Autodesk Inventor part; units mm, degrees
ref_plane "YZ Plane" through (0, 0, 0) normal (1, 0, 0) x (0, 1, 0)
ref_plane "XZ Plane" through (0, 0, 0) normal (0, 1, 0) x (-1, 0, 0)
ref_plane "XY Plane" through (0, 0, 0) normal (0, 0, 1) x (1, 0, 0)
sketch "Sketch3" plane through (0, 0, 0) normal (0, 0, 1) x (1, 0, 0)
  line L0 (0, 25.4) -> (0, -25.4)
  line L1 (0, 25.4) -> (19.05, 25.4)
  line L2 (19.05, 25.4) -> (19.05, 22.225)
  line L3 (19.05, 22.225) -> (3.048, 22.225)
  line L4 (3.048, 22.225) -> (3.048, -22.225)
  line L5 (3.048, -22.225) -> (19.05, -22.225)
  line L6 (19.05, -22.225) -> (19.05, -25.4)
  line L7 (19.05, -25.4) -> (0, -25.4)
  line L8 (0, 0) -> (3.048, 0) construction
  dimension "d7" = 50.8
  dimension "d10" = 19.05
  dimension "d19" = 3.175
  dimension "d20" = 16.002
extrude "Extrusion3" add sketch "Sketch3" along normal mid plane 209.296
fillet "Fillet1" radius 3.175 4 edges at (19.05, 22.225, 0) (19.05, -22.225, 0) (3.048, -22.225, 0) (3.048, 22.225, 0)
sketch "Sketch4" plane through (0, -25.4, 104.648) normal (-1, 0, 0) x (0, 0, 1)
  line L0 (0, 50.8) -> (-209.296, 50.8)
  line L1 (-209.296, 50.8) -> (-193.294, 50.8)
  line L2 (-193.294, 50.8) -> (-193.294, 47.625)
  line L3 (-193.294, 47.625) -> (-209.296, 47.625)
  line L4 (-209.296, 47.625) -> (-209.296, 50.8)
  line L5 (0, 44.45) -> (-209.296, 44.45)
  line L6 (-209.296, 6.35) -> (0, 6.35)
  line L7 (-209.296, 0) -> (0, 0)
  line L8 (-209.296, 0) -> (0, 0)
  line L9 (-209.296, 0) -> (-193.294, 0)
  line L10 (-193.294, 0) -> (-193.294, 3.175)
  line L11 (-193.294, 3.175) -> (-209.296, 3.175)
  line L12 (-209.296, 3.175) -> (-209.296, 0)
  line L13 (0, 3.175) -> (-209.296, 3.175)
  line L14 (-209.296, 47.625) -> (0, 47.625)
  point P0 (-104.648, 25.4)
  dimension "d14" = 16.002
extrude "Extrusion4" cut sketch "Sketch4" against normal through all
mirror "Mirror1" about plane through (0, 0, 0) normal (0, 0, 1) of "Extrusion4"
fillet "Fillet3" radius 3.175 4 edges at (3.1112, 22.225, -104.648) (3.1113, -22.225, -104.648) (3.1112, 22.225, 104.648) (3.1113, -22.225, 104.648)
equation "\"d11\" = Length"
equation "\"Length\" = 209.296"
properties part number "NASA-20-FR-BK-01" material "Aluminum 6061"
Could you check a few things on this model? Use its own coordinates, in mm. A direction names the side the tool comes from. Round coordinates to 2 decimals unless told otherwise and drop trailing zeros. Order: outer loops, then holes, each group sorted by start corner. A loop starts at its lowest first (then second) coordinate and runs counter-clockwise, first axis right, second up. Notation, with made-up numbers: M 71.5,43.5 L 82.5,43.5 A18 ccw 82.5,57.5 Z; hole C 65,58.5 d6. An arc over 180 degrees is marked long. One line per question, with ' | ' between items. Start each with the question number.
(1) Suppose I cut it at C-C on y = -13.5. List the corners of the cut face in (x, z) for me.
(2) For faces 1 (the face through (9, 25.4, -1)), 2 (the face through (3, -22.225, -95)), 3 (the face through (3.048, 0, -1)), 4 (the face through (3, 22.225, -95)), which set-ups out of +Z, -Z, +X, -X, +Y, -Y let a thin tool reach every point of the face, with its end or its side?
(3) Please list where these lines run through material, in increasing order: line 1 along Y through (x, z) = (6.25, -11.5) (3 decimals); line 2 along X through (y, z) = (4.5, 35.5); line 3 along X through (y, z) = (-19.5, 18).
(4) Suppose I cut it at B-B on x = 8.25. List the corners of the cut face in (y, z) for me (3 decimals), then the cut area to 3 significant figures.
(5) For P1, Ø1.5, axis at y = -2.5, z = -26, coming from the +X side; P2, Ø1, axis at x = 7.5, y = -23.5, coming from the +Z side; P3, Ø7, axis at x = 3, z = -98, coming from the +Y side (3 decimals), each with a flat end and sliding along its axis, tell me the tip position at first contact or that it passes through.
(6) Thinking about a two-plate mould opening in Y: for faces 5 (the face through (3, -22.225, 95)), 6 (the face through (11, 22.225, -1)), 7 (the face through (11, -22.225, -1)), 8 (the face through (3, 22.225, 95)), which applies, +Y half, -Y half, draft (parallel to the pull), parting line (faces both ways), or undercut?
Geometry results:
1) outline: M 0,-104.65 L 3.05,-104.65 L 3.05,104.65 L 0,104.65 Z
2) face 1: +Z, -Z, +X, -X, +Y | face 2: -Z, +X, -X, -Y | face 3: +Z, -Z, +X | face 4: -Z, +X, -X, +Y
3) line 1: -25.4 to -22.225, 22.225 to 25.4 | line 2: 0 to 3.05 | line 3: 0 to 3.08
4) outline: M -25.4,-88.646 L -22.225,-88.646 L -22.225,88.646 L -25.4,88.646 Z; M 22.225,-88.646 L 25.4,-88.646 L 25.4,88.646 L 22.225,88.646 Z | area: 1,130 mm²
5) P1: x = 3.05 | P2: z = 88.65 | P3: y = 22.225
6) face 5: -Y half | face 6: undercut | face 7: undercut | face 8: +Y half
